```python
from build123d import *

# Parameters (mm, degrees)
SKETCH_8_W      = 80
SKETCH_8_H      = 80
SKETCH_8_W_2    = 64
SKETCH_8_H_2    = 64
EXTRUDE_1_DEPTH = 150
SKETCH_9_W      = 120
SKETCH_9_H      = 120
SKETCH_9_R      = 12
EXTRUDE_2_DEPTH = 12
EXTRUDE_START   = 12
SKETCH_10_W     = 120
SKETCH_10_H     = 120
SKETCH_10_R     = 12
EXTRUDE_3_DEPTH = 12


with BuildPart() as part:
    # 草图8 → 凸台-拉伸1 (new, symmetric)
    with BuildSketch(Plane.XY):
        Rectangle(SKETCH_8_W, SKETCH_8_H)
        Rectangle(SKETCH_8_W_2, SKETCH_8_H_2, mode=Mode.SUBTRACT)
    extrude(amount=EXTRUDE_1_DEPTH, both=True)

    # 草图9 → 凸台-拉伸2 (add)
    with BuildSketch(Plane.XY.offset(150)):
        Rectangle(SKETCH_9_W, SKETCH_9_H)
        with Locations(Location((40, 0, 0), (0, 0, 228.189685104))):
            Circle(SKETCH_9_R, mode=Mode.SUBTRACT)
        with Locations(Location((-40, 0, 0), (0, 0, 270))):
            Circle(SKETCH_9_R, mode=Mode.SUBTRACT)
    extrude(amount=EXTRUDE_2_DEPTH)

    # 草图10 → 凸台-拉伸3 (add)
    with BuildSketch(Plane(origin=(0, 0, -150), x_dir=(-1, 0, 0), z_dir=(0, 0, -1)).offset(EXTRUDE_START)):
        Rectangle(SKETCH_10_W, SKETCH_10_H)
        with Locations(Location((40, 0, 0), (0, 0, 270))):
            Circle(SKETCH_10_R, mode=Mode.SUBTRACT)
        with Locations(Location((-40, 0, 0), (0, 0, 311.810314896))):
            Circle(SKETCH_10_R, mode=Mode.SUBTRACT)
    extrude(amount=-EXTRUDE_3_DEPTH)


solid = part.part
```
Geometry: final body of the model. Coordinates: model frame, mm. A direction names the side the tool comes from. Round coordinates to 2 decimals unless told otherwise and drop trailing zeros. Order: outer loops, then holes, each group sorted by start corner. A loop starts at its lowest first (then second) coordinate and runs counter-clockwise, first axis right, second up. Notation, with made-up numbers: (43, 54) -> (102, 54) arc R16 ccw to (102, 71) -> close; hole circle Ø3 at (-29.5, 37). An arc over 180 degrees is marked (long way). Write each question's results on one line, items separated by ' | '.
Q1. Section query B-B (x = 0). Output: boundary loops of the cut face in (y, z), and give its area (3 significant figures).
Response values:
outline: (-60, -162) -> (60, -162) -> (60, -150) -> (40, -150) -> (40, 150) -> (60, 150) -> (60, 162) -> (-60, 162) -> (-60, 150) -> (-40, 150) -> (-40, -150) -> (-60, -150) -> close; hole (-32, -150) -> (32, -150) -> (32, 150) -> (-32, 150) -> close | area: 7,680 mm²
Q2. Pin query (flat end, axial travel): pin 1 Ø1.5 at (x, z) = (-26, 113) entering from +Y; pin 2 Ø21.5 at (x, y) = (40, 0) entering from -Z; pin 3 Ø14.5 at (x, y) = (40, 0) entering from +Z. Return the tip coordinate at first contact, or that it passes through.
Response values:
pin 1: y = 40 | pin 2: z = -150 | pin 3: z = 150
Q3. Access query for faces 5 (the face through (28.157, 1.937, -156.084)), 6 (the face through (0, -32, 2)), 7 (the face through (-1, 40, 2)), 8 (the face through (40, -1, 2)), 9 (the face through (-1, -60, 156)). Directions: +Z, -Z, +X, -X, +Y, -Y. A direction counts if a zero-diameter tool reaches every point of the face in a straight line with its end or side. Return the directions, or none.
Response values:
face 5: -Z | face 6: none | face 7: +X, -X, +Y | face 8: +X, +Y, -Y | face 9: +Z, -Z, +X, -X, -Y
Q4. Ray query, line 1 along X through (y, z) = (0, 158.75); line 2 along X through (y, z) = (-28, 122); line 3 along Z through (x, y) = (52.5, 22). Return the intervals inside material, ascending.
Response values:
line 1: -60 to -52, -28 to 28, 52 to 60 | line 2: -40 to -32, 32 to 40 | line 3: -162 to -150, 150 to 162
Q5. Section query C-C (y = 0). Count the separate pieces of the cut face and the enclosed holes in it, and give its area (3 significant figures).
Response values:
separate pieces: 8 | enclosed holes: 0 | area: 6,530 mm²
Q6. Section query D-D (z = -110.5). Output: boundary loops of the cut face in (x, y).
Response values:
outline: (-40, -40) -> (40, -40) -> (40, 40) -> (-40, 40) -> close; hole (-32, -32) -> (32, -32) -> (32, 32) -> (-32, 32) -> close
Q7. Pull-direction query (Z, two-part tool) for faces 1 (the face through (-40, -1, 2)), 2 (the face through (-60, -1, -156)), 3 (the face through (36, 0, 150)), 4 (the face through (1, 1, -162)); classes: released by +Z, released by -Z, zero draft, split by the parting line, or undercut.
Response values:
face 1: undercut | face 2: zero draft | face 3: released by +Z | face 4: released by -Z
Q8. Section query A-A (y = 47). Output: boundary loops of the cut face in (x, z).
Response values:
outline: (-60, -162) -> (60, -162) -> (60, -150) -> (-60, -150) -> close; (-60, 150) -> (60, 150) -> (60, 162) -> (-60, 162) -> close
